The figure shows three views and two pictorial views of one solid part (mm, origin at its lowest corner). Answer the questions. Round coordinates to 2 decimals unless told otherwise and drop trailing zeros. Write each loop counter-clockwise with the first axis right and the second up, starting at its lowest first coordinate (ties: lowest second). Pieces come first, ordered by that corner, then holes.
Item 1: Find the intervals of material crossed by probe 1 along X at (y, z) = (0.85, 16.75); probe 2 along X at (y, z) = (2, 1.5); probe 3 along X at (y, z) = (0.95, 7.5), in increasing order.
Item 2: Find section D-D on z = 6.25. Give the vertices of the cut face in (x, y).
Item 3: Find section C-C on x = 37. Give the vertices of the cut face in (y, z).
Item 4: Find section A-A on z = 1.5. Give the vertices of the cut face in (x, y).
Item 5: Each of these flat-tipped pins is pushed along its axis until it touches: pin 1 (0.9 mm diameter, centred on y = 1.5, z = 17, fed in from +X); pin 2 (1.5 mm diameter, centred on x = 53, y = 1, fed in from +Z); pin 3 (0.9 mm diameter, centred on y = 1.5, z = 6.5, fed in from -X). Where does it stop, or does it pass through?
Item 6: Find section B-B on z = 15.5. Give the vertices of the cut face in (x, y), then the cut area to 3 significant figures.
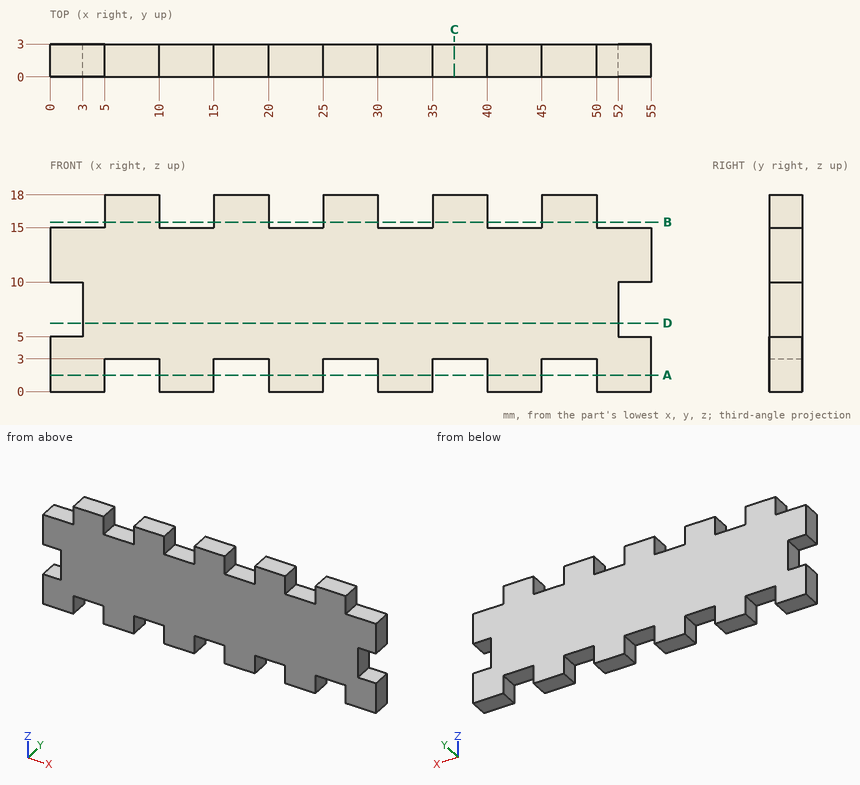
Check values:
1. probe 1: x = 5 to 10, 15 to 20, 25 to 30, 35 to 40, 45 to 50
1. probe 2: x = 0 to 5, 10 to 15, 20 to 25, 30 to 35, 40 to 45, 50 to 55
1. probe 3: x = 3 to 52
2. outline: (3, 0) - (52, 0) - (52, 3) - (3, 3) - close
3. outline: (0, 3) - (3, 3) - (3, 18) - (0, 18) - close
4. outline: (0, 0) - (5, 0) - (5, 3) - (0, 3) - close; (10, 0) - (15, 0) - (15, 3) - (10, 3) - close; (20, 0) - (25, 0) - (25, 3) - (20, 3) - close; (30, 0) - (35, 0) - (35, 3) - (30, 3) - close; (40, 0) - (45, 0) - (45, 3) - (40, 3) - close; (50, 0) - (55, 0) - (55, 3) - (50, 3) - close
5. pin 1: stops at x = 50
5. pin 2: stops at z = 15
5. pin 3: stops at x = 3
6. outline: (5, 0) - (10, 0) - (10, 3) - (5, 3) - close; (15, 0) - (20, 0) - (20, 3) - (15, 3) - close; (25, 0) - (30, 0) - (30, 3) - (25, 3) - close; (35, 0) - (40, 0) - (40, 3) - (35, 3) - close; (45, 0) - (50, 0) - (50, 3) - (45, 3) - close
6. area: 75.0 mm2
